Check sheet for the modelled part. Datum: model origin and axes. Units: mm. Round coordinates to 2 decimals unless told otherwise and drop trailing zeros. Loops run counter-clockwise (first coordinate to the right, second up) from the corner with the lowest first, then second, coordinate; pieces in that order, holes last. Notation, with made-up numbers: (40.5, 87) - (76.5, 87) arc R24 ccw to (76.5, 122) - close; hole circle Ø4 at (62.25, 47.5). An arc over 180 degrees is marked (long way). Answer in a Markdown table with one row per item. Add a question column.
(1) Cross-section at D-D on x = -15.5. Enter the section's corners in (y, z) (3 decimals).
(2) Cross-section at C-C on y = 21.5. Enter the section's corners in (x, z) (3 decimals).
(3) Thickness scan on line 1 along Y through (x, z) = (-35, -2.55); line 2 along Y through (x, z) = (-36.83, -1.9); line 3 along X through (y, z) = (9, -2.05). Record the ranges inside material, lowest first.
(4) Gauge pin test, flat ends, axial feed: pin 1 (1 mm diameter, centred on x = -41, z = -1, fed in from -Y); pin 2 (1.5 mm diameter, centred on x = -16.5, z = -2, fed in from +Y). Record the tip position at first contact, or that the pin passes through.
(5) Cross-section at B-B on z = -0.5. Count the separate pieces of the cut face and the enclosed holes in it, then the cut area to 3 significant figures.
(6) Cross-section at A-A on y = 88. Enter the section's corners in (x, z) (3 decimals), then the cut area to 3 significant figures.
from build123d import *

# Parameters (mm, degrees)
BOSS_EXTRUDE1_DEPTH             = 3.175
F_6_CLEARANCE_HOLE1_D           = 4.3053
F_1_2_0_5_DIAMETER_HOLE1_D      = 12.7
F_9_64_0_14063_DIAMETER_HOLE1_D = 3.572002


with BuildPart() as part:
    # Sketch1 → Boss-Extrude1 (new body)
    with BuildSketch(Plane.XY):
        with BuildLine():
            Line((-25.4, 0), (0, 0))
            Line((0, 0), (0, 130.81))
            Line((0, 130.81), (-9.144, 130.81))
            Line((-9.144, 130.81), (-45.72, 101.6))
            Line((-45.72, 101.6), (-45.72, 22.86))
            Line((-45.72, 22.86), (-28.575, 22.86))
            ThreePointArc((-28.575, 22.86), (-26.32993597, 21.93006403), (-25.4, 19.685))
            Line((-25.4, 19.685), (-25.4, 0))
        make_face()
    extrude(amount=-BOSS_EXTRUDE1_DEPTH)

    # #6 Clearance Hole1 (through all)
    with Locations(Plane.XY):
        with Locations((-5.715, 34.925), (-36.83, 33.3375), (-5.715, 121.158)):
            Hole(F_6_CLEARANCE_HOLE1_D / 2)

    # 1/2 (0.5) Diameter Hole1 (through all)
    with Locations(Plane.XY):
        with Locations((-25.4, 83.058)):
            Hole(F_1_2_0_5_DIAMETER_HOLE1_D / 2)

    # 9/64 (0.14063) Diameter Hole1 (through all)
    with Locations(Plane.XY):
        with Locations((-25.4, 73.533)):
            Hole(F_9_64_0_14063_DIAMETER_HOLE1_D / 2)


solid = part.part
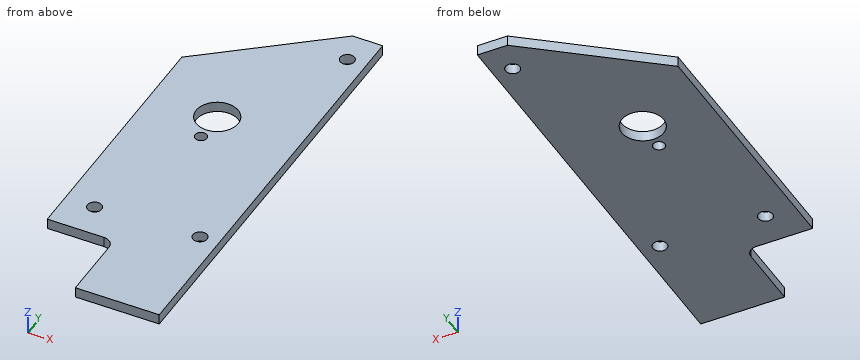
Answers:
| question | item | result |
|---|---|---|
| 1 | outline | (0, -3.175) - (125.734, -3.175) - (125.734, 0) - (0, 0) - close |
| 2 | outline | (-25.97, -3.175) - (0, -3.175) - (0, 0) - (-25.97, 0) - close |
| 3 | line 1 | y = 22.86 to 32.2, 34.47 to 110.16 |
| 3 | line 2 | y = 22.86 to 31.18, 35.49 to 108.7 |
| 3 | line 3 | x = -25.4 to 0 |
| 4 | pin 1 | stops at y = 22.86 |
| 4 | pin 2 | stops at y = 125.53 |
| 5 | separate pieces | 1 |
| 5 | enclosed holes | 5 |
| 5 | area | 4,800 mm^2 |
| 6 | outline | (-45.72, -3.175) - (-29.387, -3.175) - (-29.387, 0) - (-45.72, 0) - close; (-21.413, -3.175) - (0, -3.175) - (0, 0) - (-21.413, 0) - close |
| 6 | area | 120 mm^2 |
